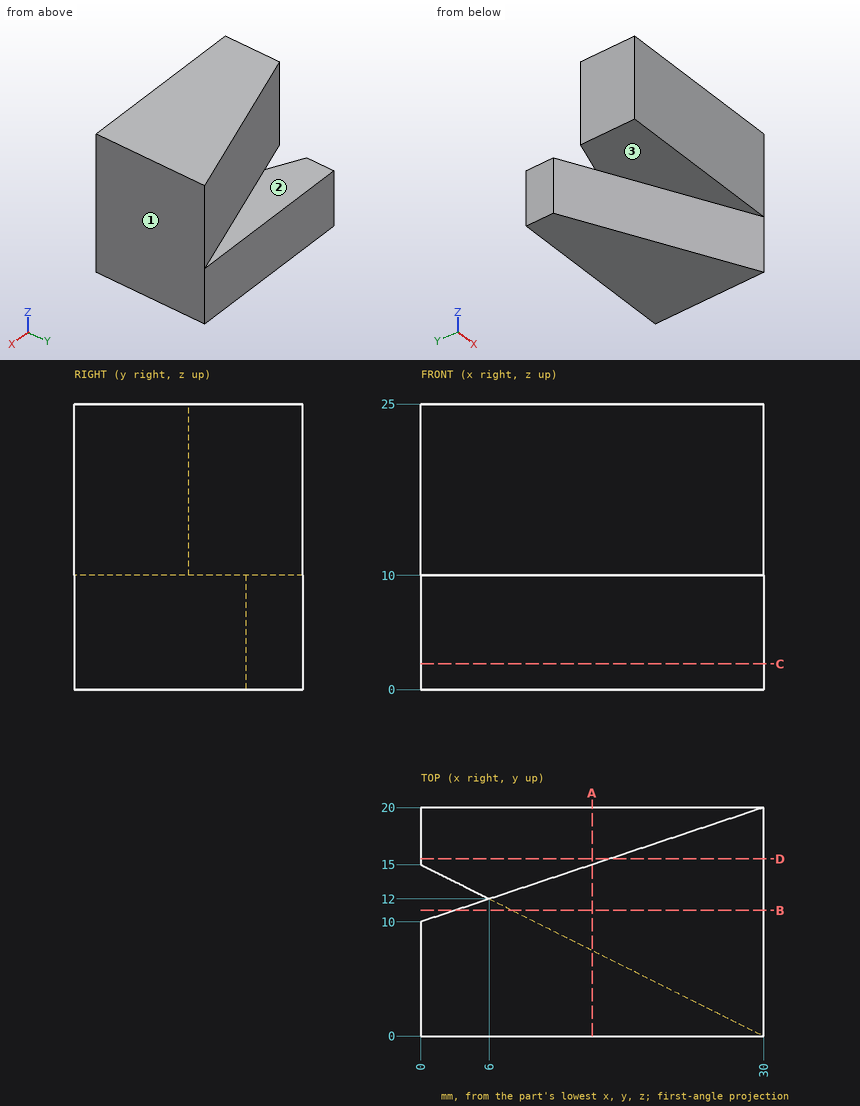
Source: three-view drawing plus pictorial views. Frame: mm from the lowest corner of the part. A direction names the side the tool comes from. Coordinates: 2 decimals unless noted, no trailing zeros. Order: outer loops, then holes, each group sorted by start corner. A loop starts at its lowest first (then second) coordinate and runs counter-clockwise, first axis right, second up. Notation, with made-up numbers: M 75.25,7 L 125.25,7 A24 cw 125.25,31 Z; hole C -6,72.25 d2. An arc over 180 degrees is marked long. One line per question, with ' | ' between items. Start each with the question number.
Item 1: Cut plane B-B, the plane y = 11. Return the cut outline in (x, z), then the cut area to 3 significant figures.
Item 2: Cut plane D-D, the plane y = 15.5. Return the cut outline in (x, z), then the cut area to 4 significant figures.
Item 3: Cut plane C-C, the plane z = 2.25. Return the cut outline in (x, y), then the cut area to 3 significant figures.
Item 4: Pin query (flat end, axial travel): pin 1 Ø4 at (x, z) = (16, 7.5) entering from -Y; pin 2 Ø3.5 at (x, y) = (9.5, 6.5) entering from -Z; pin 3 Ø3 at (y, z) = (2, 6) entering from -X. Return the tip coordinate at first contact, or that it passes through.
Item 5: Set-up query: the marked faces 1, 2 and 3. Return all of +Z, -Z, +X, -X, +Y, -Y with unobstructed straight access to the full face (end or side cutting, diameter ignored); none if empty.
Item 6: Ray query, probe 1 along Z at (x, y) = (15.5, 15.5); probe 2 along Z at (x, y) = (18, 5.75); probe 3 along Y at (x, z) = (8, 2). Return the intervals inside material, ascending. Write a range as [from, to].
Item 7: Cut plane A-A, the plane x = 15. Return the cut outline in (y, z), then the cut area to 3 significant figures.
A:
1) outline: M 3,10 L 8,10 L 8,0 L 30,0 L 30,25 L 3,25 Z | area: 625 mm2
2) outline: M 0,0 L 30,0 L 30,25 L 16.5,25 L 16.5,10 L 0,10 Z | area: 502.5 mm2
3) outline: M 0,15 L 30,0 L 30,20 L 0,20 Z | area: 375 mm2
4) pin 1: stops at y = 6 | pin 2: stops at z = 10 | pin 3: stops at x = 23
5) face 1: +Z, -Z, +X, +Y, -Y | face 2: +Z, -X, +Y | face 3: -Z, -X, -Y
6) probe 1: z = [0, 10] | probe 2: z = [10, 25] | probe 3: y = [11, 20]
7) outline: M 0,10 L 7.5,10 L 7.5,0 L 20,0 L 20,10 L 15,10 L 15,25 L 0,25 Z | area: 350 mm2
